Check sheet for the modelled part. Datum: model origin and axes. Units: mm. Round coordinates to 2 decimals unless told otherwise and drop trailing zeros. Loops run counter-clockwise (first coordinate to the right, second up) from the corner with the lowest first, then second, coordinate; pieces in that order, holes last. Notation, with made-up numbers: (40, -1) -> (84, -1) arc R17 ccw to (84, 10) -> close; hole circle Ø4 at (-17, -19). An arc over 180 degrees is marked (long way). Return JSON: item names as keys, results as strings.
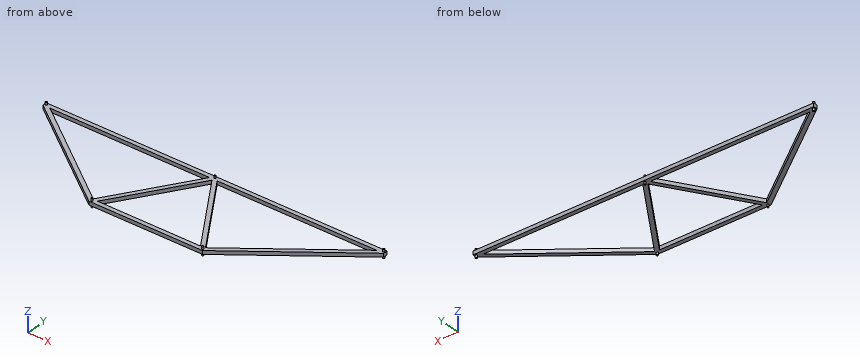
from build123d import *

# Parameters (mm, degrees)
BOSS_EXTRUDE2_DEPTH = 6.375
SKETCH3_R           = 3.3
BOSS_EXTRUDE3_DEPTH = 14.975


with BuildPart() as part:
    # Sketch1 → Boss-Extrude2 (new, symmetric)
    with BuildSketch(Plane.XY):
        Polygon((0, -7.245), (0, 0), (-600, 0), (-600, -14.49), (-591.306, -2.898), (-575.85, -14.49), (-13.344393946, -14.49), (-6.075978819, -3.298798486), align=None)
        Polygon((0, -20.546405114), (-3.933488865, -14.49), (-13.344393946, -14.49), (-197.595006689, -298.181244983), (-195.17, -300), (-181.498361341, -300), align=None)
        Polygon((-575.85, -14.49), (-600, -14.49), (-200, -314.49), (-200, -307.806399497), (-202.705205395, -306.049433921), (-200, -301.884220709), (-200, -300), (-198.776244152, -300), (-197.595006689, -298.181244983), align=None)
        Polygon((13.344393946, -14.49), (3.933488865, -14.49), (0, -20.546405114), (181.498361341, -300), (195.17, -300), (197.595006689, -298.181244983), align=None)
        Polygon((600, 0), (0, 0), (0, -7.245), (6.075978819, -3.298798486), (13.344393946, -14.49), (575.85, -14.49), (591.306, -2.898), (600, -14.49), align=None)
        Polygon((200, -314.49), (600, -14.49), (575.85, -14.49), (197.595006689, -298.181244983), (198.776244152, -300), (200, -300), (200, -301.884220709), (202.705205395, -306.049433921), (200, -307.806399497), align=None)
        Polygon((-200, -314.49), (200, -314.49), (196.629226576, -309.995635435), (190.553247757, -313.941836949), (181.498361341, -300), (-181.498361341, -300), (-190.553247757, -313.941836949), (-196.629226576, -309.995635435), align=None)
        Polygon((6.075978819, -3.298798486), (0, -7.245), (6.075978819, -11.191201514), (3.933488865, -14.49), (13.344393946, -14.49), align=None)
        Polygon((-6.075978819, -11.191201514), (0, -7.245), (-6.075978819, -3.298798486), (-13.344393946, -14.49), (-3.933488865, -14.49), align=None)
        Polygon((6.075978819, -11.191201514), (0, -7.245), (0, -14.49), (3.933488865, -14.49), align=None)
        Polygon((0, -14.49), (0, -7.245), (-6.075978819, -11.191201514), (-3.933488865, -14.49), align=None)
        Polygon((3.933488865, -14.49), (0, -14.49), (-3.933488865, -14.49), (0, -20.546405114), align=None)
        Polygon((198.776244152, -300), (197.595006689, -298.181244983), (195.17, -300), align=None)
        Polygon((200, -300), (198.776244152, -300), (200, -301.884220709), align=None)
        Polygon((200, -301.884220709), (200, -307.806399497), (202.705205395, -306.049433921), align=None)
        Polygon((196.629226576, -309.995635435), (200, -314.49), (200, -307.806399497), align=None)
        Polygon((196.629226576, -309.995635435), (200, -307.806399497), (200, -301.884220709), (198.776244152, -300), (195.17, -300), (191.306, -302.898), align=None)
        Polygon((190.553247757, -313.941836949), (196.629226576, -309.995635435), (191.306, -302.898), (195.17, -300), (181.498361341, -300), align=None)
        Polygon((575.85, -14.49), (600, -14.49), (591.306, -2.898), align=None)
        Polygon((-591.306, -2.898), (-600, -14.49), (-575.85, -14.49), align=None)
        Polygon((-191.306, -302.898), (-196.629226576, -309.995635435), (-190.553247757, -313.941836949), (-181.498361341, -300), (-195.17, -300), align=None)
        Polygon((-200, -307.806399497), (-200, -314.49), (-196.629226576, -309.995635435), align=None)
        Polygon((-202.705205395, -306.049433921), (-200, -307.806399497), (-200, -301.884220709), align=None)
        Polygon((-195.17, -300), (-197.595006689, -298.181244983), (-198.776244152, -300), align=None)
        Polygon((-200, -301.884220709), (-198.776244152, -300), (-200, -300), align=None)
        Polygon((-200, -301.884220709), (-200, -307.806399497), (-196.629226576, -309.995635435), (-191.306, -302.898), (-195.17, -300), (-198.776244152, -300), align=None)
    extrude(amount=BOSS_EXTRUDE2_DEPTH, both=True)

    # Sketch3 → Boss-Extrude3 (add, symmetric)
    with BuildSketch(Plane.XY):
        with Locations((0, -7.245)):
            Circle(SKETCH3_R)
        with Locations((-194.842755286, -307.245)):
            Circle(SKETCH3_R)
        with Locations((194.842755286, -307.245)):
            Circle(SKETCH3_R)
        with Locations((594.56625, -7.245)):
            Circle(SKETCH3_R)
        with Locations((-594.56625, -7.245)):
            Circle(SKETCH3_R)
    extrude(amount=BOSS_EXTRUDE3_DEPTH, both=True)


solid = part.part
Q1. Section check D-D (x = -137). Record the boundary of the cut face in (y, z) (3 decimals), then the cut area to 3 significant figures.
Results list:
{"outline": "(-314.49, -6.375) -> (-300, -6.375) -> (-300, 6.375) -> (-314.49, 6.375) -> close; (-231.486, -6.375) -> (-204.883, -6.375) -> (-204.883, 6.375) -> (-231.486, 6.375) -> close; (-14.49, -6.375) -> (0, -6.375) -> (0, 6.375) -> (-14.49, 6.375) -> close", "area": "709 mm^2"}
Q2. Go/stop test with flat-tipped pins: pin 1 (5 mm diameter, centred on y = -153.5, z = -1, fed in from +X); pin 2 (10 mm diameter, centred on x = 256.5, z = -1, fed in from -Y) (3 decimals); pin 3 (10 mm diameter, centred on x = -1.5, z = 10, fed in from +Y); pin 4 (6 mm diameter, centred on x = 269.5, z = 0, fed in from -Y) (3 decimals). Record where each tip stops, or that it passes through.
Results list:
{"pin 1": "x = 417.99", "pin 2": "y = -275.865", "pin 3": "y = 0", "pin 4": "y = -264.615"}
Q3. Section check C-C (y = -71). Record the boundary of the cut face in (x, z) (3 decimals).
Results list:
{"outline": "(-524.653, -6.375) -> (-500.503, -6.375) -> (-500.503, 6.375) -> (-524.653, 6.375) -> close; (-50.046, -6.375) -> (-32.768, -6.375) -> (-32.768, 6.375) -> (-50.046, 6.375) -> close; (32.768, -6.375) -> (50.046, -6.375) -> (50.046, 6.375) -> (32.768, 6.375) -> close; (500.503, -6.375) -> (524.653, -6.375) -> (524.653, 6.375) -> (500.503, 6.375) -> close"}
Q4. Section check A-A (z = 0.75). Record the boundary of the cut face in (x, y) (3 decimals).
Results list:
{"outline": "(-600, -14.49) -> (-200, -314.49) -> (200, -314.49) -> (600, -14.49) -> (600, 0) -> (-600, 0) -> close; hole (-575.85, -14.49) -> (-197.595, -298.181) -> (-13.344, -14.49) -> close; hole (-181.498, -300) -> (181.498, -300) -> (0, -20.546) -> close; hole (13.344, -14.49) -> (197.595, -298.181) -> (575.85, -14.49) -> close"}
Q5. Material ranges on line 1 (Y direction, x = -109, z = -0.25); line 2 (X direction, y = -161, z = 2.25); line 3 (X direction, y = -130, z = -6.25), recorded low to high.
Results list:
{"line 1": "-314.49 to -300, -188.37 to -161.77, -14.49 to 0", "line 2": "-404.65 to -380.5, -108.5 to -91.22, 91.22 to 108.5, 380.5 to 404.65", "line 3": "-445.99 to -421.84, -88.37 to -71.09, 71.09 to 88.37, 421.84 to 445.99"}
Q6. Section check B-B (x = 348). Record the boundary of the cut face in (y, z) (1 decimal), then the cut area to 3 significant figures.
Results list:
{"outline": "(-203.5, -6.4) -> (-185.4, -6.4) -> (-185.4, 6.4) -> (-203.5, 6.4) -> close; (-14.5, -6.4) -> (0, -6.4) -> (0, 6.4) -> (-14.5, 6.4) -> close", "area": "416 mm^2"}
